Geometry: final body of the model. Coordinates: model frame, mm. A direction names the side the tool comes from. Give positions to 0.01 mm unless a question says otherwise; leave off trailing zeros. Write each loop counter-clockwise with the first axis right and the second up, starting at its lowest first coordinate (ties: lowest second). Pieces come first, ordered by that corner, then holes. Notation, with made-up numbers: (64, 79) -> (76, 79) arc R26 cw to (76, 103) -> close; hole circle Ø10 at (67.5, 82.5). An arc over 180 degrees is marked (long way). Answer as a JSON object with one key per item and string values. Group by question number.
(1) Set-up query: faces 4 (the face through (-15, 1.5, 14)), 5 (the face through (0, 0, 0)). Return all of +Z, -Z, +X, -X, +Y, -Y with unobstructed straight access to the full face (end or side cutting, diameter ignored); none if empty.
(2) Section query C-C on z = -14.25. Output: boundary loops of the cut face in (x, y), plus the area to 4 significant figures.
(3) Section query B-B on x = 0. Output: boundary loops of the cut face in (y, z).
(4) Section query D-D on z = -6.5. Output: boundary loops of the cut face in (x, y).
(5) Contact query for a flat-ended pin moving along its axis: pin 1 Ø18 at (x, z) = (-8.5, 2) entering from +Y. Output: stop coordinate, or through.
(6) Section query A-A on y = 4.5. State how many separate pieces and enclosed holes the cut face has, plus the area to 3 significant figures.
(7) Material intervals for probe 1 along X at (y, z) = (7.5, -14.25); probe 2 along Z at (x, y) = (-11.5, 5.25); probe 3 along X at (y, z) = (6.5, -15), sorted ascending.
(8) Draft query along Z for faces 1 (the face through (-14.35, 5.69, 15.36)), 2 (the face through (16, 10, -15)), 3 (the face through (17.795, 3.451, 20.896)). Return one class per face: +Z half, -Z half, draft (parallel to the pull), parting line (faces both ways), or undercut.
from build123d import *

# Parameters (mm, degrees)
SKETCH_1_W           = 36.5
SKETCH_1_H           = 42.5
EXTRUDE_1_DEPTH      = 1.5
FILLET_1_R           = 5
SKETCH_2_R           = 1.4
SKETCH_2_R_2         = 0.85
EXTRUDE_2_DEPTH      = 8.5
EXTRUDE_3_DEPTH      = 5.5
EXTRUDE_3_DEPTH_BACK = 1.5


with BuildPart() as part:
    # 草图1 → 凸台-拉伸1 (new body)
    with BuildSketch(Plane(origin=(0, 0, 0), x_dir=(1, 0, 0), z_dir=(0, 1, 0))):
        Rectangle(SKETCH_1_W, SKETCH_1_H)
    extrude(amount=EXTRUDE_1_DEPTH)

    # 圆角1
    fillet_1_edges = [part.edges().sort_by_distance(p)[0] for p in [
        (18.25, 0.75, 21.25),
        (-18.25, 0.75, 21.25),
        (-18.25, 0.75, -21.25),
        (18.25, 0.75, -21.25),
    ]]
    fillet(fillet_1_edges, radius=FILLET_1_R)

    # 草图2 → 凸台-拉伸2 (add)
    # profile 1 of 4: a face of its own
    with BuildSketch(Plane(origin=(0, 1.5, 0), x_dir=(1, 0, 0), z_dir=(0, 1, 0))):
        with Locations(Location((-15.2, 14.25, 0), (0, 0, 270))):
            Circle(SKETCH_2_R)
        with Locations(Location((-15.2, 14.25, 0), (0, 0, 270))):
            Circle(SKETCH_2_R_2, mode=Mode.SUBTRACT)
    # profile 2 of 4: a face of its own
    with BuildSketch(Plane(origin=(0, 1.5, 0), x_dir=(1, 0, 0), z_dir=(0, 1, 0))):
        with Locations(Location((-15.2, -14.25, 0), (0, 0, 90))):
            Circle(SKETCH_2_R)
        with Locations(Location((-15.2, -14.25, 0), (0, 0, 90))):
            Circle(SKETCH_2_R_2, mode=Mode.SUBTRACT)
    # profile 3 of 4: a face of its own
    with BuildSketch(Plane(origin=(0, 1.5, 0), x_dir=(1, 0, 0), z_dir=(0, 1, 0))):
        with Locations(Location((15.2, -14.25, 0), (0, 0, 270))):
            Circle(SKETCH_2_R)
        with Locations(Location((15.2, -14.25, 0), (0, 0, 270))):
            Circle(SKETCH_2_R_2, mode=Mode.SUBTRACT)
    # profile 4 of 4: a face of its own
    with BuildSketch(Plane(origin=(0, 1.5, 0), x_dir=(1, 0, 0), z_dir=(0, 1, 0))):
        with Locations(Location((15.2, 14.25, 0), (0, 0, 90))):
            Circle(SKETCH_2_R)
        with Locations(Location((15.2, 14.25, 0), (0, 0, 90))):
            Circle(SKETCH_2_R_2, mode=Mode.SUBTRACT)
    extrude(amount=EXTRUDE_2_DEPTH)

    # 草图3 → 凸台-拉伸3 (add, two sides: drawn at the far end of the back side and taken through both)
    with BuildSketch(Plane(origin=(0, 1.5, 0), x_dir=(1, 0, 0), z_dir=(0, 1, 0)).offset(-EXTRUDE_3_DEPTH_BACK)):
        with BuildLine():
            Line((-13.25, -22.75), (13.25, -22.75))
            ThreePointArc((13.25, -22.75), (17.846194078, -20.846194078), (19.75, -16.25))
            Line((19.75, -16.25), (19.75, 16.25))
            ThreePointArc((19.75, 16.25), (17.846194078, 20.846194078), (13.25, 22.75))
            Line((13.25, 22.75), (-13.25, 22.75))
            ThreePointArc((-13.25, 22.75), (-17.846194078, 20.846194078), (-19.75, 16.25))
            Line((-19.75, 16.25), (-19.75, -16.25))
            ThreePointArc((-19.75, -16.25), (-17.846194078, -20.846194078), (-13.25, -22.75))
        make_face()
        with BuildLine():
            Line((-13.25, -21.25), (13.25, -21.25))
            ThreePointArc((13.25, -21.25), (16.785533906, -19.785533906), (18.25, -16.25))
            Line((18.25, -16.25), (18.25, 16.25))
            ThreePointArc((18.25, 16.25), (16.785533906, 19.785533906), (13.25, 21.25))
            Line((13.25, 21.25), (-13.25, 21.25))
            ThreePointArc((-13.25, 21.25), (-16.785533906, 19.785533906), (-18.25, 16.25))
            Line((-18.25, 16.25), (-18.25, -16.25))
            ThreePointArc((-18.25, -16.25), (-16.785533906, -19.785533906), (-13.25, -21.25))
        make_face(mode=Mode.SUBTRACT)
    extrude(amount=EXTRUDE_3_DEPTH + EXTRUDE_3_DEPTH_BACK)


solid = part.part
Answer list:
{
 "1": {"face 4": "+Y", "face 5": "+Z, -Z, +X, -X, -Y"},
 "2": {"outline": "(-19.75, 0) -> (19.75, 0) -> (19.75, 7) -> (18.25, 7) -> (18.25, 1.5) -> (16.6, 1.5) -> (16.6, 10) -> (16.05, 10) -> (16.05, 1.5) -> (14.35, 1.5) -> (14.35, 10) -> (13.8, 10) -> (13.8, 1.5) -> (-13.8, 1.5) -> (-13.8, 10) -> (-14.35, 10) -> (-14.35, 1.5) -> (-16.05, 1.5) -> (-16.05, 10) -> (-16.6, 10) -> (-16.6, 1.5) -> (-18.25, 1.5) -> (-18.25, 7) -> (-19.75, 7) -> close", "area": "94.45 mm2"},
 "3": {"outline": "(0, -22.75) -> (7, -22.75) -> (7, -21.25) -> (1.5, -21.25) -> (1.5, 21.25) -> (7, 21.25) -> (7, 22.75) -> (0, 22.75) -> close"},
 "4": {"outline": "(-19.75, 0) -> (19.75, 0) -> (19.75, 7) -> (18.25, 7) -> (18.25, 1.5) -> (-18.25, 1.5) -> (-18.25, 7) -> (-19.75, 7) -> close"},
 "5": {"pin 1": "y = 1.5"},
 "6": {"separate pieces": "5", "enclosed holes": "5", "area": "247 mm2"},
 "7": {"probe 1": "-16.6 to -16.05, -14.35 to -13.8, 13.8 to 14.35, 16.05 to 16.6", "probe 2": "-22.75 to -21.25, 21.25 to 22.75", "probe 3": "-19.75 to -18.25, -16.38 to -15.6, -14.8 to -14.02, 14.02 to 14.8, 15.6 to 16.38, 18.25 to 19.75"},
 "8": {"face 1": "undercut", "face 2": "draft", "face 3": "+Z half"}
}
